Can you work these out from the model? Positions are in its coordinate system, mm. A direction names the side the tool comes from. Give positions to 0.01 mm unless a question says otherwise; leave off trailing zeros. Loops run counter-clockwise (first coordinate to the right, second up) from the corner with the lowest first, then second, coordinate; pieces in that order, holes last. Notation, with made-up numbers: (49.5, 69.5) -> (53.5, 69.5) arc R24 ccw to (53.5, 91.5) -> close; hole circle Ø11 at (-4, 76.5). An arc over 180 degrees is marked (long way). Use CSV: the item, a comma, the result in double quotes.
from build123d import *
from build123d.topology import SkipClean

# Parameters (mm, degrees)
REVOLVE_4_ANGLE     = 180.0000000000004
SKETCH_2_W          = 15.068111951450035
SKETCH_2_H          = 7.96575550760617
CUT_EXTRUDE_1_DEPTH = 56.00000000000002
SKETCH_3_R          = 4.999999999999991
EXTRUDE_2_DEPTH     = 43.00000000000001
SKETCH_45_R         = 8.000000000000014
CUT_EXTRUDE_2_DEPTH = 10
REVOLVE_5_ANGLE     = 180.0000000000004


with BuildPart() as part:
    # 草图1 → 旋转4 (revolve)
    with BuildSketch(Plane.XY):
        with BuildLine():
            Line((110.00000000000001, 81.99999999999996), (110.00000000000001, 89.99999999999999))
            Line((110.00000000000001, 89.99999999999999), (110.00000000000001, 98))
            ThreePointArc((110.00000000000001, 98), (102, 89.99999999999999), (110.00000000000001, 81.99999999999997))
        make_face()
    revolve(axis=Axis((110.00000000000001, 81.99999999999996, 0), (0, 1, 0)), revolution_arc=REVOLVE_4_ANGLE)

    # 草图2 → 切除-拉伸1 (cut)
    with SkipClean():  # the faces are left unmerged after this step: merging them gives an invalid solid
        with BuildSketch(Plane(origin=(0, 119.99999999999999, 0), x_dir=(1, 0, 0), z_dir=(0, 1, 0))):
            with Locations((110, -6.673230993554715)):
                Rectangle(SKETCH_2_W, SKETCH_2_H)
        extrude(amount=-CUT_EXTRUDE_1_DEPTH, mode=Mode.SUBTRACT)

    # 草图45 → 切除-拉伸2 (cut)
    with BuildSketch(Plane(origin=(0, 0, 0), x_dir=(-1, 0, 6.98e-15), z_dir=(-6.98e-15, 0, -1))):
        with Locations((-110.00000000000001, 89.99999999999999)):
            Circle(SKETCH_45_R)
    extrude(amount=-CUT_EXTRUDE_2_DEPTH, mode=Mode.SUBTRACT)


with BuildPart() as body_2:
    # 草图3 → 凸台-拉伸2 (new body)
    with BuildSketch(Plane(origin=(0, 0, 0), x_dir=(-1, 0, 6.98e-15), z_dir=(-6.98e-15, 0, -1))):
        with Locations((-117.96224151764466, 79.27742160371339)):
            Circle(SKETCH_3_R)
    extrude(amount=EXTRUDE_2_DEPTH)

    # 草图46 → 旋转5 (revolve)
    with BuildSketch(Plane.XY):
        with BuildLine():
            ThreePointArc((117.96224151764446, 74.2774216037134), (112.96224151764467, 79.2774216037134), (117.96224151764447, 84.27742160371338))
            Line((117.96224151764436, 84.27742160371338), (117.96224151764436, 86.27742160371339))
            ThreePointArc((117.96224151764436, 86.27742160371339), (110.96224151764436, 79.27742160371339), (117.96224151764436, 72.27742160371339))
            Line((117.96224151764436, 72.27742160371338), (117.96224151764436, 74.2774216037134))
        make_face()
        with BuildLine():
            Line((117.96224151764436, 74.2774216037134), (117.96224151764436, 79.27742160371339))
            Line((117.96224151764436, 79.27742160371339), (117.96224151764436, 84.27742160371338))
            ThreePointArc((117.96224151764447, 84.27742160371338), (112.96224151764467, 79.2774216037134), (117.96224151764446, 74.2774216037134))
        make_face()
        with BuildLine():
            Line((117.96224151764436, 84.27742160371338), (117.96224151764436, 79.27742160371339))
            Line((117.96224151764436, 79.27742160371339), (117.96224151764436, 74.2774216037134))
            ThreePointArc((117.96224151764446, 74.2774216037134), (121.49777542357731, 75.74188769778058), (122.96224151764464, 79.27742160371339))
            ThreePointArc((122.96224151764464, 79.27742160371339), (121.49777542357732, 82.81295550964619), (117.96224151764447, 84.27742160371338))
        make_face()
    revolve(axis=Axis((117.96224151764436, 86.27742160371339, 0), (0, 1, 0)), revolution_arc=REVOLVE_5_ANGLE)


solid = body_2.part
(1) If we section it at B-B, the plane x = 115.25: Write out the boundary of the cut face in (y, z).
Answer sheet:
outline,"(72.82, 0) -> (75.08, 0) -> (75.08, -43) -> (83.48, -43) -> (83.48, 0) -> (85.73, 0) arc R6.45 ccw to start"
(2) If we section it at C-C, the plane z = -27.5: Write out the boundary of the cut face in (x, y).
Answer sheet:
outline,"circle Ø10 at (117.96, 79.28)"
(3) Which directions (+Z, -Z, +X, -X, +Y, -Y) give clear straight access to the entire face, cutting with the end or side of a thin tool? Please do faces 1 (the face through (113, 81, 0)), 2 (the face through (118, 79, -43)).
Answer sheet:
face 1,"-Z"
face 2,"-Z, +X, -X, +Y, -Y"
(4) If I drill on L1, parallel to Y at x = 118, z = -14; L2, parallel to Z at x = 116.25, y = 74.75; L3, parallel to Z at x = 114, y = 83.25, over which ranges is the centre line in solid material (lowest first)? Write a range as from..to.
Answer sheet:
L1,"y = 74.28..84.28"
L2,"z = -43..5.06"
L3,"z = 0..4.19"
(5) Will these pins go through, and if not, where does the flat tip stop? pin 1 Ø8 at (x, y) = (114.5, 83.5) entering from +Z; pin 2 Ø1 at (y, z) = (81.5, -17.5) entering from +X; pin 3 Ø4 at (x, z) = (114, -14.5) entering from +Y.
Answer sheet:
pin 1,"stops at z = 6.85"
pin 2,"stops at x = 122.66"
pin 3,"stops at y = 83.88"
(6) If we section it at A-A, the plane y = 78.75: Write out the boundary of the cut face in (x, z), then the cut area to 3 significant figures.
Answer sheet:
outline,"(110.98, 0) -> (112.99, 0) -> (112.99, -43) -> (122.93, -43) -> (122.93, 0) -> (124.94, 0) arc R6.98 ccw to start"
area,"504 mm2"
